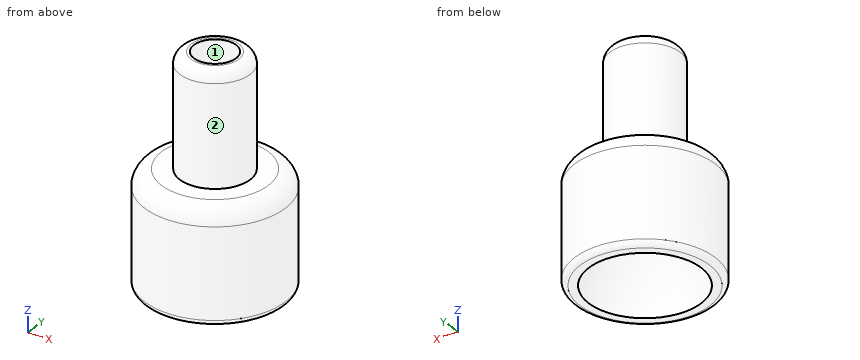
```python
from build123d import *


with BuildPart() as f1:
    # F0 (on Front) → F1 (revolve)
    with BuildSketch(Plane.XZ):
        with BuildLine():
            Line((-15.875, 22.86), (-15.875, 2.54))
            ThreePointArc((-15.875, 2.54), (-15.503026, 1.641974), (-14.605, 1.27))
            Line((-14.605, 1.27), (-12.7, 1.27))
            add(Edge.make_bspline(
                [(-4.7625, 24.587877), (-4.910941, 17.2893), (-12.796914, 11.896686), (-12.7, 1.27)],
                knots=[0, 0, 0, 0, 24.631835, 24.631835, 24.631835, 24.631835], degree=3))
            Line((-4.7625, 24.587877), (-4.7625, 52.07))
            Line((-4.7625, 52.07), (-5.3975, 52.07))
            ThreePointArc((-5.3975, 52.07), (-7.193551, 51.326051), (-7.9375, 49.53))
            Line((-7.9375, 49.53), (-7.9375, 26.67))
            Line((-7.9375, 26.67), (-12.065, 26.67))
            ThreePointArc((-12.065, 26.67), (-14.759077, 25.554077), (-15.875, 22.86))
        make_face()
    revolve(axis=Axis((0, 0, 25.536608), (0, 0, 1)))


solid = f1.part
```
Geometry: final body of the model. Coordinates: model frame, mm. Face numbers are marked on the shaded views. A direction names the side the tool comes from. Give positions to 0.01 mm unless a question says otherwise; leave off trailing zeros. Write each loop counter-clockwise with the first axis right and the second up, starting at its lowest first coordinate (ties: lowest second). Pieces come first, ordered by that corner, then holes.
1. Section query A-A, the plane z = 35. Return loops of the section in (x, y) (1 decimal).
2. Reachability of the marked faces 1 and 2 from +Z, -Z, +X, -X, +Y, -Y: full face, straight path, thin tool, end or side. Return the list, or none.
3. Pin query (flat end, axial travel): P1, Ø8, axis at x = -2.5, y = 6, coming from the -Z side; P2, Ø12, axis at y = -4.5, z = 34.5, coming from the +X side; P3, Ø6, axis at x = 11.5, y = 4, coming from the +Z side. Return the tip coordinate at first contact, or that it passes through.
4. Line query: probe 1 along X at (y, z) = (0, 36.25); probe 2 along X at (y, z) = (-2.5, 42.5). Output: solid intervals per line, ascending.
Computed:
1. outline: circle Ø15.9 at (0, 0); hole circle Ø9.5 at (0, 0)
2. face 1: +Z, -Z
2. face 2: +Z
3. P1: stops at z = 10.9
3. P2: stops at x = 7.94
3. P3: stops at z = 26.67
4. probe 1: x = -7.94 to -4.76, 4.76 to 7.94
4. probe 2: x = -7.53 to -4.05, 4.05 to 7.53
